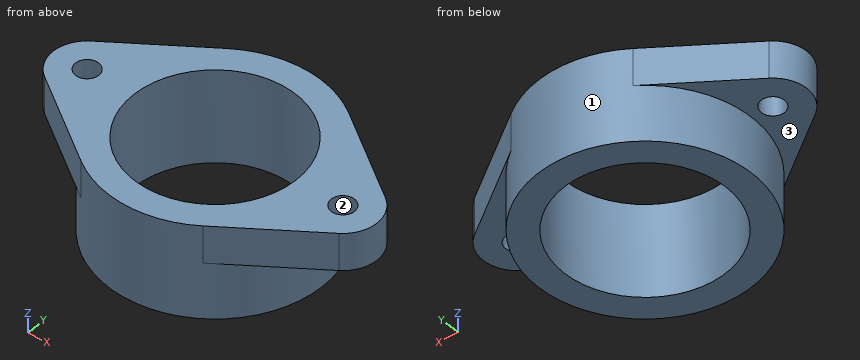
Autodesk Inventor part; units mm, degrees
ref_plane "YZ Plane" through (0, 0, 0) normal (1, 0, 0) x (0, 1, 0)
ref_plane "XZ Plane" through (0, 0, 0) normal (0, 1, 0) x (-1, 0, 0)
ref_plane "XY Plane" through (0, 0, 0) normal (0, 0, 1) x (1, 0, 0)
sketch "スケッチ1" plane through (0, 0, 0) normal (0, 0, 1) x (1, 0, 0)
  circle A0 centre (0, 0) radius 2.25 construction
  circle A1 centre (0, 0) radius 4.35
  circle A2 centre (0, 0) radius 5.75
  circle A3 centre (-6.875, 0) radius 0.625
  circle A4 centre (6.875, 0) radius 0.625
  circle A5 centre (0, 0) radius 6.875 construction
  circle A6 centre (-6.875, 0) radius 1.825
  circle A7 centre (6.875, 0) radius 1.825
  line L0 (-7.9169, 1.4983) -> (-3.2827, 4.7208)
  line L1 (-7.9169, -1.4983) -> (-3.2827, -4.7208)
  line L2 (7.9169, -1.4983) -> (3.2827, -4.7208)
  line L3 (3.2827, 4.7208) -> (7.9169, 1.4983)
  line L4 (6.875, 0) -> (0, 0) construction
  line L5 (0, 0) -> (-6.875, 0) construction
  circle A8 centre (0, 0) radius 4.25
  point P0 (5.5998, -1.3056)
  point P1 (5.5998, 1.3056)
  point P2 (-5.5998, 1.3056)
  point P3 (-5.5998, -1.3056)
  dimension "d2" = 4.5
  dimension "d5" = 1.25
  dimension "d6" = 1.25
  dimension "d7" = 1.2
  dimension "d8" = 1.2
  dimension "d9" = 0.5
  dimension "d18" = 180
  dimension "d22" = 13.75
  dimension "d23" = 0.1
  dimension "d24" = 8.5
  dimension "d25" = 1.5
extrude "押し出し1" add sketch "スケッチ1" against normal blind 5 contours A2 A7 A6 | A2 A7 | A6 A2 picked at (5.515, -0.2153) picked at (-5.5055, 0)
extrude "押し出し3" add sketch "スケッチ1" against normal blind 2 contours A2 A6 L0 | A2 A6 | A2 L1 A6 picked at (-5.951, -0.7528)
extrude "押し出し4" add sketch "スケッチ1" against normal blind 2 contours L3 A7 A2 | A7 A2 | A7 L2 A2 picked at (6.0448, 0.9837)
equation "\"d6\" = d5"
equation "\"d8\" = d7"
properties part number "motorauxiliary"
Design review of the part built by this model. Coordinates are the model's own, in mm. Face numbers are marked on the shaded views. Coordinates: 2 decimals unless noted, no trailing zeros. Order: outer loops, then holes, each group sorted by start corner. A loop starts at its lowest first (then second) coordinate and runs counter-clockwise, first axis right, second up.
1) Take a section at C-C, the plane y = 0. Give the boundary of the cut face in (x, z).
2) Take a section at A-A, the plane x = 0. Give the boundary of the cut face in (y, z).
3) Wall thickness on line 1 along Y through (x, z) = (0, -1.25); line 2 along X through (y, z) = (-3.75, -4.5); line 3 along X through (y, z) = (-1.75, -3.05): over which ranges is each line inside the solid? List them lowest first.
4) Take a section at D-D, the plane z = -4.05. Give the boundary of the cut face in (x, y), and give its area (3 significant figures).
5) Take a section at B-B, the plane y = 2.5. Give the boundary of the cut face in (x, z).
6) Mouldability with a two-part tool opening along X and no side actions: class the marked faces 1, 2 and 3 as +X half, -X half, draft (parallel to the pull), parting line (faces both ways), or undercut.
7) Clearance check with flat-ended pins moving along their axes: pin 1 (3 mm diameter, centred on x = 6.5, z = -4, fed in from -Y); pin 2 (1.1 mm diameter, centred on x = 6.875, y = 0, fed in from +Z); pin 3 (1.5 mm diameter, centred on y = 4, z = -1, fed in from +X). State where each tip first meets the part, or that it passes through.
Returned:
1. outline: (-8.7, -2) - (-7.5, -2) - (-7.5, 0) - (-8.7, 0) - close; (-6.25, -2) - (-5.75, -2) - (-5.75, -5) - (-4.35, -5) - (-4.35, 0) - (-6.25, 0) - close; (4.35, -5) - (5.75, -5) - (5.75, -2) - (6.25, -2) - (6.25, 0) - (4.35, 0) - close; (7.5, -2) - (8.7, -2) - (8.7, 0) - (7.5, 0) - close
2. outline: (-5.75, -5) - (-4.35, -5) - (-4.35, 0) - (-5.75, 0) - close; (4.35, -5) - (5.75, -5) - (5.75, 0) - (4.35, 0) - close
3. line 1: y = -5.75 to -4.35, 4.35 to 5.75
3. line 2: x = -4.36 to -2.2, 2.2 to 4.36
3. line 3: x = -5.48 to -3.98, 3.98 to 5.48
4. outline: circle Ø11.5 at (0, 0); hole circle Ø8.7 at (0, 0)
4. area: 44.4 mm2
5. outline: (-6.48, -2) - (-5.18, -2) - (-5.18, -5) - (-3.56, -5) - (-3.56, 0) - (-6.48, 0) - close; (3.56, -5) - (5.18, -5) - (5.18, -2) - (6.48, -2) - (6.48, 0) - (3.56, 0) - close
6. face 1: parting line
6. face 2: undercut
6. face 3: draft
7. pin 1: stops at y = -2.84
7. pin 2: passes through
7. pin 3: stops at x = 5.4
